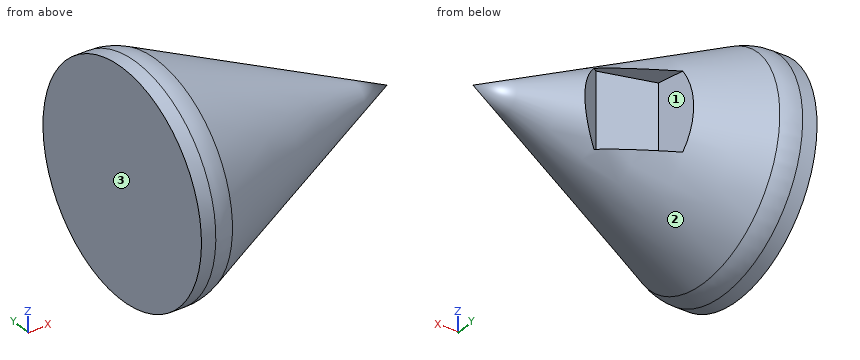
Autodesk Fusion 360 part; units mm, degrees
sketch "Sketch1" plane through (0, 0, 0) normal (0, 1, 0) x (1, 0, 0)
  line L0 (0, 0) -> (272, 0)
  line L1 (0, 0) -> (0, -115)
  line L2 (0, -115) -> (14.7579, -115)
  line L3 (35.0449, -110.5022) -> (272, 0)
  arc A0 (14.7579, -115) -> (35.0449, -110.5022) centre (14.7579, -67) ccw
  point P0 (25.4, -115)
  dimension "d1" = 272
  dimension "d2" = 115
  dimension "d3" = 25.4
  dimension "d4" = 48
revolve "Revolve1" add sketch "Sketch1" angle 360 about axis through (0, 0, 0) along (1, 0, 0)
ref_plane "WorkPlane1" through (0, 0, 0) normal (0, 0, 1) x (1, 0, 0)
sketch "Sketch2" plane through (0, 0, 0) normal (0, 0, 1) x (1, 0, 0)
  line L0 (100.5395, 84.3629) -> (110, 40)
  line L1 (110, 40) -> (163.6315, 25.2684)
  line L2 (163.6315, 25.2684) -> (189.7167, 43.1547)
  line L3 (189.7167, 43.1547) -> (100.5395, 84.3629)
extrude "Extrude1" cut sketch "Sketch2" along normal mid plane 80
Check sheet for the modelled part. Datum: model origin and axes. Units: mm. Face numbers are marked on the shaded views. Coordinates: 2 decimals unless noted, no trailing zeros. Write each loop counter-clockwise with the first axis right and the second up, starting at its lowest first coordinate (ties: lowest second). Pieces come first, ordered by that corner, then holes.
Item 1: Mould release check, pull along Z, two halves, no side actions. Record for the marked faces 1, 2 and 3: released by +Z, released by -Z, zero draft, split by the parting line, or undercut.
Numbers:
face 1: undercut
face 2: split by the parting line
face 3: zero draft
Item 2: Cross-section at A-A on x = 228.5. Record the boundary of the cut face in (y, z), then the cut area to 3 significant figures.
Numbers:
outline: circle Ø40.57 at (0, 0)
area: 1,290 mm2
Item 3: Depth check by flat-ended pin: pin 1 Ø3 at (y, z) = (28.5, 64) entering from +X; pin 2 Ø12.5 at (x, y) = (123.5, 48.5) entering from -Z; pin 3 Ø6 at (y, z) = (-17.5, 23.5) entering from +X. Enter the tip coordinate at first touch or a pass-through.
Numbers:
pin 1: stops at x = 124.99
pin 2: stops at z = -56.11
pin 3: stops at x = 215.6
Item 4: Cross-section at B-B on x = 26.5. Record the boundary of the cut face in (y, z), then the cut area to 3 significant figures.
Numbers:
outline: circle Ø227.08 at (0, 0)
area: 40,500 mm2
Item 5: Scan lines: probe 1 along Z at (x, y) = (35.5, 12.5); probe 2 along X at (y, z) = (-55.5, -77.5); probe 3 along X at (y, z) = (56, 23.5). Record each from-to range of solid material in increasing order.
Numbers:
probe 1: z = -109.58 to 109.58
probe 2: x = 0 to 67.59
probe 3: x = 0 to 106.59
Item 6: Cross-section at C-C on x = 135.5. Record the boundary of the cut face in (y, z).
Numbers:
outline: (33, -40) - (33, 40) - (49.52, 40) arc R63.66 ccw (long way) to (49.52, -40) - close
